Geometry check sheet. Reference: the model listing, model coordinates, mm. A direction names the side the tool comes from. Give positions to 0.01 mm unless a question says otherwise; leave off trailing zeros. Write each loop counter-clockwise with the first axis right and the second up, starting at its lowest first coordinate (ties: lowest second). Pieces come first, ordered by that corner, then holes. Notation, with made-up numbers: (5, -3) -> (19, -3) arc R30 ccw to (19, 30) -> close; hole circle Ø3 at (73.5, 10). An arc over 180 degrees is marked (long way). One line per item, written item: value.
Autodesk Inventor part; units mm, degrees
ref_plane "YZ Plane" through (0, 0, 0) normal (1, 0, 0) x (0, 1, 0)
ref_plane "XZ Plane" through (0, 0, 0) normal (0, 1, 0) x (-1, 0, 0)
ref_plane "XY Plane" through (0, 0, 0) normal (0, 0, 1) x (1, 0, 0)
sketch "草圖1" plane through (0, 0, 0) normal (0, 1, 0) x (-1, 0, 0)
  line L0 (-33.5, 27) -> (33.5, 27)
  line L1 (33.5, 27) -> (33.5, -27)
  line L2 (33.5, -27) -> (-33.5, -27)
  line L3 (-33.5, -27) -> (-33.5, 27)
  line L4 (-33.5, 27) -> (33.5, -27) construction
  line L5 (33.5, 27) -> (-33.5, -27) construction
  line L6 (43.5, -4.5) -> (33.5, -4.5)
  line L7 (33.5, -4.5) -> (33.5, 4.5)
  line L8 (33.5, 4.5) -> (43.5, 4.5)
  line L9 (43.5, 4.5) -> (43.5, -4.5)
  line L10 (-33.5, -4.5) -> (-43.5, -4.5)
  line L11 (-43.5, -4.5) -> (-43.5, 4.5)
  line L12 (-43.5, 4.5) -> (-33.5, 4.5)
  line L13 (-33.5, 4.5) -> (-33.5, -4.5)
  point P0 (0, 0)
  point P1 (33.5, 0)
  point P2 (-33.5, 0)
  point P3 (-33.5, 4.5)
  point P4 (-33.5, -4.5)
  dimension "d0" = 67
  dimension "d1" = 54
  dimension "d2" = 9
  dimension "d3" = 10
extrude "擠出1" add sketch "草圖1" along normal blind 350
sketch "草圖2" plane through (-33.5, 0, 27) normal (0, 0, 1) x (1, 0, 0)
  line L0 (0, 0) -> (0, 350)
  line L1 (0, 350) -> (67, 350)
  line L2 (67, 350) -> (67, 0)
  line L3 (67, 0) -> (0, 0)
  circle A0 centre (33.5, 148) radius 30
  line L4 (3.5, 148) -> (63.5, 148)
  line L5 (63.5, 148) -> (63.5, -3.654)
  line L6 (63.5, -3.654) -> (3.5, -3.654)
  line L7 (3.5, -3.654) -> (3.5, 148)
  point P0 (33.5, 0)
  point P1 (33.5, 0)
  point P2 (63.5, 148)
  point P3 (3.5, 148)
  dimension "d6" = 148
  dimension "d7" = 60
extrude "擠出2" cut sketch "草圖2" against normal through all contours L7 A0 L5 L3 | L3 L5 L6 L7 | L4 A0 | A0 L4
sketch "草圖3" plane through (-33.5, 350, 27) normal (0, 0, 1) x (1, 0, 0)
  line L0 (-135.2961, -270) -> (202.2961, -270)
  line L1 (202.2961, -270) -> (202.2961, -350)
  line L2 (202.2961, -350) -> (-135.2961, -350)
  line L3 (-135.2961, -350) -> (-135.2961, -270)
  point P0 (33.5, -350)
  point P1 (33.5, -350)
  dimension "d10" = 80
extrude "擠出3" cut sketch "草圖3" against normal through all
sketch "草圖4" plane through (33.5, 350, -27) normal (0, 0, -1) x (-1, 0, 0)
  arc A0 (63.5, -202) -> (3.5, -202) centre (33.5, -202) ccw construction
  circle A1 centre (33.5, -182) radius 30
  line L0 (63.5, -270) -> (3.5, -270)
  line L1 (3.5, -270) -> (3.5, -182)
  line L2 (3.5, -182) -> (63.5, -182)
  line L3 (63.5, -182) -> (63.5, -270)
  line L4 (63.5, -270) -> (67, -270)
  point P0 (33.5, -350)
  point P1 (65.25, -270)
  dimension "d13" = 20
  dimension "d14" = 60
sketch "草圖5" plane through (-33.5, 350, 27) normal (0, 0, 1) x (1, 0, 0)
  arc A0 (63.5, -202) -> (3.5, -202) centre (33.5, -202) ccw construction
  circle A1 centre (33.5, -180) radius 30
  line L0 (63.5, -270) -> (3.5, -270)
  line L1 (3.5, -270) -> (3.5, -180)
  line L2 (3.5, -180) -> (63.5, -180)
  line L3 (63.5, -180) -> (63.5, -270)
  point P0 (33.5, -350)
  point P1 (63.5, -270)
  dimension "d15" = 22
  dimension "d16" = 60
loft "斷面混成1" cut profiles "草圖4", "草圖5"
properties part number "Slider-6"
1) Mould release check, pull along X, two halves, no side actions. Record for faces 1 (the flat face through (-33.5, 213, -16)), 2 (the flat face through (43.5, 213, 0)), 3 (the flat face through (30, 126, 0)): released by +X, released by -X, zero draft, split by the parting line, or undercut.
Verdict:
face 1: released by -X
face 2: released by +X
face 3: undercut
2) Scan lines: probe 1 along X at (y, z) = (108, -1); probe 2 along X at (y, z) = (169, -16); probe 3 along X at (y, z) = (216.5, -19.5). Record each from-to range of solid material in increasing order.
Verdict:
probe 1: -43.5 to -30, 30 to 43.5
probe 2: -33.5 to -29.99, 29.99 to 33.5
probe 3: -33.5 to 33.5
3) Sectioned sample at A-A on y = 118. Record the cut outline in (x, z).
Verdict:
outline: (-43.5, -4.5) -> (-33.5, -4.5) -> (-33.5, -27) -> (-30, -27) -> (-30, 27) -> (-33.5, 27) -> (-33.5, 4.5) -> (-43.5, 4.5) -> close; (30, -27) -> (33.5, -27) -> (33.5, -4.5) -> (43.5, -4.5) -> (43.5, 4.5) -> (33.5, 4.5) -> (33.5, 27) -> (30, 27) -> close
4) Depth check by flat-ended pin: pin 1 Ø5 at (x, y) = (39.5, 224.5) entering from +Z; pin 2 Ø3 at (x, y) = (40.5, 259.5) entering from -Z; pin 3 Ø7 at (y, z) = (264, 13) entering from -X; pin 4 Ø8 at (x, y) = (-36.5, 212.5) entering from +Z. Enter the tip coordinate at first touch or a pass-through.
Verdict:
pin 1: z = 4.5
pin 2: z = -4.5
pin 3: x = -33.5
pin 4: z = 27
5) Sectioned sample at B-B on y = 210. Record the cut outline in (x, z), plus the area to 3 significant figures.
Verdict:
outline: (-43.5, -4.5) -> (-33.5, -4.5) -> (-33.5, -27) -> (33.5, -27) -> (33.5, -4.5) -> (43.5, -4.5) -> (43.5, 4.5) -> (33.5, 4.5) -> (33.5, 27) -> (-33.5, 27) -> (-33.5, 4.5) -> (-43.5, 4.5) -> close
area: 3,800 mm^2
6) Sectioned sample at C-C on x = -37. Record the cut outline in (y, z).
Verdict:
outline: (80, -4.5) -> (350, -4.5) -> (350, 4.5) -> (80, 4.5) -> close
7) Tool access check on faces 4 (the flat face through (38, 213, -4.5)), 5 (the flat face through (33.5, 213, 16)), 6 (the flat face through (-30, 124, 0)), 7 (the flat face through (-39, 213, -4.5)), 8 (the flat face through (-38, 213, 4.5)). Record the directions out of +Z, -Z, +X, -X, +Y, -Y that give a thin tool (end or side, any length) a straight path to the whole face; none if there is none.
Verdict:
face 4: -Z, +X, +Y, -Y
face 5: +Z, +X, +Y, -Y
face 6: +Z, -Z, -Y
face 7: -Z, -X, +Y, -Y
face 8: +Z, -X, +Y, -Y
